Could you check a few things on this model? Use its own coordinates, in mm. Face numbers are marked on the shaded views. A direction names the side the tool comes from. Give positions to 0.01 mm unless a question says otherwise; leave off trailing zeros. Write each loop counter-clockwise with the first axis right and the second up, starting at its lowest first coordinate (ties: lowest second). Pieces come first, ordered by that corner, then holes. Notation, with made-up numbers: (26, -36) - (46, -36) arc R32 cw to (46, -6) - close; hole circle Ø11 at (78.5, 55). An arc over 180 degrees is marked (long way). Answer in a Markdown table with one row per item.
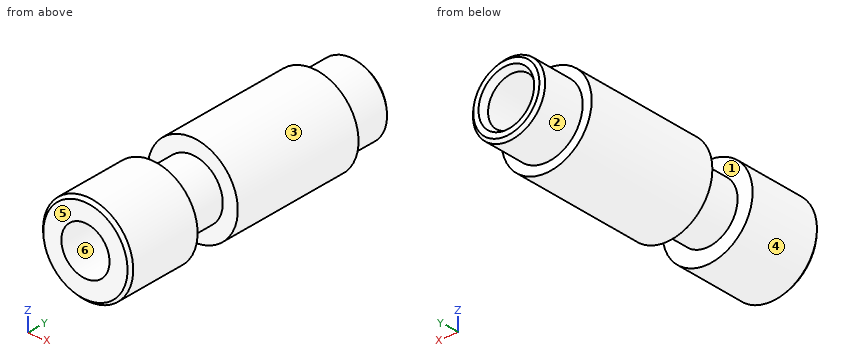
from build123d import *

# Parameters (mm, degrees)
CHAFL_N4_SIZE  = 0.2
CHAFL_N5_SIZE  = 0.25
CHAFL_N5_SIZE2 = 0.433012702


with BuildPart() as part:
    # Croquis3 → Revolución1 (revolve)
    with BuildSketch(Plane.XY):
        Polygon((-1.6, 0), (-1.6, 20), (-2.4, 20), (-2.4, 17), (-3, 17), (-3, 8), (-2, 8), (-2, 5), (-3, 5), (-3, 0), align=None)
    revolve(axis=Axis((0, 0, 0), (0, 1, 0)))

    # Chaflán4
    chafl_n4_edges = [part.edges().sort_by_distance(p)[0] for p in [
        (2.4, 20, 0),
        (3, 0, 0),
    ]]
    chamfer(chafl_n4_edges, length=CHAFL_N4_SIZE)

    # Chaflán5
    chafl_n5_edges = [part.edges().sort_by_distance(p)[0] for p in [
        (1.6, 20, 0),
    ]]
    chafl_n5_side = [part.faces().sort_by_distance(p)[0] for p in [
        (2.137774603, 20, 0),
    ]]
    chamfer(chafl_n5_edges, length=CHAFL_N5_SIZE, length2=CHAFL_N5_SIZE2, reference=chafl_n5_side[0])


solid = part.part
1) If I drill on line 1 (Z direction, x = 0, y = 12.5); line 2 (Y direction, x = 2.25, z = 1); line 3 (Y direction, x = 1.3, z = -1.65), over which ranges is the centre line in solid material (lowest first)?
Check values:
| item | result |
|---|---|
| line 1 | z = -3 to -1.6, 1.6 to 3 |
| line 2 | y = 0 to 5, 8 to 17 |
| line 3 | y = 0 to 5, 8 to 20 |
2) Will these pins go through, and if not, where does the flat tip stop? P1, Ø2, axis at x = -2, y = 12.5, coming from the +Z side; P2, Ø3, axis at x = 0.5, z = -1, coming from the +Y side.
Check values:
| item | result |
|---|---|
| P1 | stops at z = 2.83 |
| P2 | stops at y = 20 |
3) We'd pull the mould along Z, two halves only. Please class the marked faces 4, 5 and 6: +Z half, -Z half, draft (parallel to the pull), parting line (faces both ways), or undercut.
Check values:
| item | result |
|---|---|
| face 4 | parting line |
| face 5 | draft |
| face 6 | undercut |
4) On a 3-axis mill with a long thin cutter (end or side, diameter ignored), from which of +Z, -Z, +X, -X, +Y, -Y can I reach the whole of each face in a straight line? I mean the marked faces 1, 2 and 3. Say none if no direction works.
Check values:
| item | result |
|---|---|
| face 1 | none |
| face 2 | +Y |
| face 3 | +Y, -Y |
5) Imagine slicing it at B-B (x = 0). List the corners of the cut face in (y, z) for me.
Check values:
| item | result |
|---|---|
| outline | (0, -2.8) - (0.2, -3) - (5, -3) - (5, -2) - (8, -2) - (8, -3) - (17, -3) - (17, -2.4) - (19.8, -2.4) - (20, -2.2) - (20, -1.85) - (19.57, -1.6) - (0, -1.6) - close; (0, 1.6) - (19.57, 1.6) - (20, 1.85) - (20, 2.2) - (19.8, 2.4) - (17, 2.4) - (17, 3) - (8, 3) - (8, 2) - (5, 2) - (5, 3) - (0.2, 3) - (0, 2.8) - close |
6) Imagine slicing it at C-C (y = 13). List the corners of the cut face in (x, z) for me, then the cut area to 3 significant figures.
Check values:
| item | result |
|---|---|
| outline | circle Ø6 at (0, 0); hole circle Ø3.2 at (0, 0) |
| area | 20.2 mm2 |
7) Imagine slicing it at A-A (z = 0). List the corners of the cut face in (x, y) for me, then the cut area to 3 significant figures.
Check values:
| item | result |
|---|---|
| outline | (-3, 0.2) - (-2.8, 0) - (-1.6, 0) - (-1.6, 19.57) - (-1.85, 20) - (-2.2, 20) - (-2.4, 19.8) - (-2.4, 17) - (-3, 17) - (-3, 8) - (-2, 8) - (-2, 5) - (-3, 5) - close; (1.6, 0) - (2.8, 0) - (3, 0.2) - (3, 5) - (2, 5) - (2, 8) - (3, 8) - (3, 17) - (2.4, 17) - (2.4, 19.8) - (2.2, 20) - (1.85, 20) - (1.6, 19.57) - close |
| area | 46.2 mm2 |
